```python
from build123d import *

# Parameters (mm, degrees)
F2_W      = 457.2
F2_H      = 304.8
F3_DEPTH  = 12.7
F4_W      = 431.8
F4_H      = 20.0152
F5_DEPTH  = 6.35
F7_D      = 3.3
F8_R      = 2.3876
F9_DEPTH  = 6.35
F10_W     = 6.35
F10_H     = 283.6672
F11_DEPTH = 1.5875


# Not quite as in the source:
# - a variable given as a bare number and used for a length is read in inches; the dataset says mm whatever the document's units were


with BuildPart() as f3:
    # F2 (on Top) → F3 (new body)
    with BuildSketch(Plane.XY):
        Rectangle(F2_W, F2_H)
    extrude(amount=F3_DEPTH)

    # F4 (on face) → F5 (cut)
    with BuildSketch(Plane.XY.offset(12.7)):
        with Locations((0, 131.826)):
            Rectangle(F4_W, F4_H)
        with Locations((0, 105.4608)):
            Rectangle(F4_W, F4_H)
        with Locations((0, 79.0956)):
            Rectangle(F4_W, F4_H)
        with Locations((0, 52.7304)):
            Rectangle(F4_W, F4_H)
        with Locations((0, 26.3652)):
            Rectangle(F4_W, F4_H)
        Rectangle(F4_W, F4_H)
        with Locations((0, -26.3652)):
            Rectangle(F4_W, F4_H)
        with Locations((0, -52.7304)):
            Rectangle(F4_W, F4_H)
        with Locations((0, -79.0956)):
            Rectangle(F4_W, F4_H)
        with Locations((0, -105.4608)):
            Rectangle(F4_W, F4_H)
        with Locations((0, -131.826)):
            Rectangle(F4_W, F4_H)
    extrude(amount=-F5_DEPTH, mode=Mode.SUBTRACT)

    # F7 (through all)
    with Locations(Plane.XY.offset(12.7)):
        with Locations((-223.3168, 147.1168), (-223.3168, 73.5584), (-223.3168, 0), (-223.3168, -73.5584), (-223.3168, -147.1168), (-148.8778666667, -147.1168), (-74.4389333333, -147.1168), (0, -147.1168), (74.4389333333, -147.1168), (148.8778666667, -147.1168), (223.3168, -147.1168), (223.3168, -73.5584), (223.3168, 0), (223.3168, 73.5584), (223.3168, 147.1168), (148.8778666667, 147.1168), (74.4389333333, 147.1168), (0, 147.1168), (-74.4389333333, 147.1168), (-148.8778666667, 147.1168)):
            Hole(F7_D / 2)

    # F8 (on face) → F9 (cut)
    with BuildSketch(Plane.XY.offset(12.7)):
        with Locations((-215.9, 33.9852)):
            Circle(F8_R)
        with Locations((-215.9, 45.1104)):
            Circle(F8_R)
        with Locations((-215.9, 60.3504)):
            Circle(F8_R)
        with Locations((-215.9, 86.7156)):
            Circle(F8_R)
        with Locations((-215.9, 71.4756)):
            Circle(F8_R)
        with Locations((-215.9, 97.8408)):
            Circle(F8_R)
        with Locations((-215.9, 113.0808)):
            Circle(F8_R)
        with Locations((-215.9, 124.206)):
            Circle(F8_R)
        with Locations((-215.9, 139.446)):
            Circle(F8_R)
        with Locations((-215.9, 18.7452)):
            Circle(F8_R)
        with Locations((-215.9, 7.62)):
            Circle(F8_R)
        with Locations((215.9, 7.62)):
            Circle(F8_R)
        with Locations((215.9, 18.7452)):
            Circle(F8_R)
        with Locations((215.9, 33.9852)):
            Circle(F8_R)
        with Locations((215.9, 45.1104)):
            Circle(F8_R)
        with Locations((215.9, 60.3504)):
            Circle(F8_R)
        with Locations((215.9, 71.4756)):
            Circle(F8_R)
        with Locations((215.9, 86.7156)):
            Circle(F8_R)
        with Locations((215.9, 97.8408)):
            Circle(F8_R)
        with Locations((215.9, 113.0808)):
            Circle(F8_R)
        with Locations((215.9, 124.206)):
            Circle(F8_R)
        with Locations((215.9, 139.446)):
            Circle(F8_R)
        with Locations((215.9, -7.62)):
            Circle(F8_R)
        with Locations((215.9, -18.7452)):
            Circle(F8_R)
        with Locations((215.9, -33.9852)):
            Circle(F8_R)
        with Locations((215.9, -45.1104)):
            Circle(F8_R)
        with Locations((215.9, -60.3504)):
            Circle(F8_R)
        with Locations((215.9, -71.4756)):
            Circle(F8_R)
        with Locations((215.9, -86.7156)):
            Circle(F8_R)
        with Locations((215.9, -97.8408)):
            Circle(F8_R)
        with Locations((215.9, -113.0808)):
            Circle(F8_R)
        with Locations((215.9, -124.206)):
            Circle(F8_R)
        with Locations((215.9, -139.446)):
            Circle(F8_R)
        with Locations((-215.9, -7.62)):
            Circle(F8_R)
        with Locations((-215.9, -18.7452)):
            Circle(F8_R)
        with Locations((-215.9, -33.9852)):
            Circle(F8_R)
        with Locations((-215.9, -45.1104)):
            Circle(F8_R)
        with Locations((-215.9, -60.3504)):
            Circle(F8_R)
        with Locations((-215.9, -71.4756)):
            Circle(F8_R)
        with Locations((-215.9, -97.8408)):
            Circle(F8_R)
        with Locations((-215.9, -86.7156)):
            Circle(F8_R)
        with Locations((-215.9, -139.446)):
            Circle(F8_R)
        with Locations((-215.9, -124.206)):
            Circle(F8_R)
        with Locations((-215.9, -113.0808)):
            Circle(F8_R)
    extrude(amount=-F9_DEPTH, mode=Mode.SUBTRACT)

    # F10 (on face) → F11 (cut)
    with BuildSketch(Plane.XY.offset(12.7)):
        Rectangle(F10_W, F10_H)
    extrude(amount=-F11_DEPTH, mode=Mode.SUBTRACT)


solid = f3.part
```
Input: part model. Units: mm. Frame: model coordinates. A direction names the side the tool comes from. Coordinates: 2 decimals unless noted, no trailing zeros.
1) Pin query (flat end, axial travel): pin 1 Ø4 at (x, y) = (-223.32, 0) entering from +Z; pin 2 Ø10 at (x, y) = (-76.5, 51) entering from +Z. Return the tip coordinate at first contact, or that it passes through.
2) Set-up query: faces 1 (the flat face through (-3, 2, 0)), 2 (the flat face through (-3, 132, 6.35)). Return all of +Z, -Z, +X, -X, +Y, -Y with unobstructed straight access to the full face (end or side cutting, diameter ignored); none if empty.
3) Section A-A on z = 8.5. State how many separate pieces and enclosed holes the cut face has, and give its area (3 significant figures).
4) Mould query, pull axis X, two halves, no side actions, for faces 3 (the flat face through (-228.6, -2, 6)), 4 (the flat face through (-3, -53, 6.35)), 5 (the flat face through (-3, -152.4, 6)), 6 (the flat face through (-3, 27, 6.35)). Classes: pulls with the +X half, pulls with the -X half, needs draft (parallel to the pull), parting line crosses it, or undercut.
5) Material intervals for line 1 along X through (y, z) = (-38, 11.5) (3 decimals); line 2 along X through (y, z) = (76.5, 6.5); line 3 along Z through (x, y) = (-156.5, -123), sorted ascending.
Check result:
1. pin 1: stops at z = 12.7
1. pin 2: stops at z = 6.35
2. face 1: -Z, +X, -X, +Y, -Y
2. face 2: +Z
3. separate pieces: 1
3. enclosed holes: 31
3. area: 43,700 mm2
4. face 3: pulls with the -X half
4. face 4: undercut
4. face 5: needs draft
4. face 6: undercut
5. line 1: x = -228.6 to -3.175, 3.175 to 228.6
5. line 2: x = -228.6 to -215.9, 215.9 to 228.6
5. line 3: z = 0 to 6.35
